```python
from build123d import *

# Parameters (mm, degrees)
BOSS_EXTRUDE2_DEPTH = 26
SKETCH5_R           = 1.6
CUT_EXTRUDE4_DEPTH  = 26
SKETCH6_R           = 1.6
CUT_EXTRUDE6_DEPTH  = 26


with BuildPart() as part:
    # Sketch1 → Boss-Extrude2 (new body)
    with BuildSketch(Plane(origin=(0, 0, 0), x_dir=(1, 0, 0), z_dir=(0, 1, 0))):
        Polygon((-24.25, 0), (24.25, 0), (24.25, -11), (39.25, -11), (39.25, -6), (29.25, -6), (29.25, 5), (5, 5), (5, 10), (-5, 10), (-5, 5), (-29.25, 5), (-29.25, -6), (-39.25, -6), (-39.25, -11), (-24.25, -11), align=None)
    extrude(amount=BOSS_EXTRUDE2_DEPTH)

    # Sketch5 → Cut-Extrude4 (cut)
    with BuildSketch(Plane.XZ):
        with Locations(Location((0, -5, 0), (0, 0, 270))):
            Circle(SKETCH5_R)
    extrude(amount=-CUT_EXTRUDE4_DEPTH, mode=Mode.SUBTRACT)

    # Sketch6 → Cut-Extrude6 (cut)
    with BuildSketch(Plane(origin=(0, 0, 6), x_dir=(-1, 0, 0), z_dir=(0, 0, -1))):
        with Locations((34.25, 19.5)):
            Circle(SKETCH6_R)
        with Locations((34.25, 6.5)):
            Circle(SKETCH6_R)
        with Locations((-34.25, 6.5)):
            Circle(SKETCH6_R)
        with Locations((-34.25, 19.5)):
            Circle(SKETCH6_R)
    extrude(amount=-CUT_EXTRUDE6_DEPTH, mode=Mode.SUBTRACT)


solid = part.part
```
Design review of the part built by this model. Coordinates are the model's own, in mm. A direction names the side the tool comes from. Give positions to 0.01 mm unless a question says otherwise; leave off trailing zeros. Write each loop counter-clockwise with the first axis right and the second up, starting at its lowest first coordinate (ties: lowest second). Pieces come first, ordered by that corner, then holes.
(1) Clearance check with flat-ended pins moving along their axes: pin 1 Ø3.5 at (x, y) = (34.25, 19.5) entering from +Z; pin 2 Ø5 at (x, y) = (32, 11.5) entering from -Z; pin 3 Ø3 at (x, y) = (-12.5, 7.5) entering from +Z; pin 4 Ø7.5 at (x, y) = (-13.5, 6.5) entering from -Z. State where each tip first meets the part, or that it passes through.
Checked values:
pin 1: stops at z = 11
pin 2: stops at z = 6
pin 3: stops at z = 0
pin 4: stops at z = -5
(2) Add section D-D (y = 3.5). Give the boundary of the cut face in (x, z), and give its area (3 significant figures).
Checked values:
outline: (-39.25, 6) - (-29.25, 6) - (-29.25, -5) - (-5, -5) - (-5, -10) - (5, -10) - (5, -5) - (29.25, -5) - (29.25, 6) - (39.25, 6) - (39.25, 11) - (24.25, 11) - (24.25, 0) - (-24.25, 0) - (-24.25, 11) - (-39.25, 11) - close; hole circle Ø3.2 at (0, -5)
area: 544 mm2
(3) Add section A-A (y = 19.5). Give the boundary of the cut face in (x, z), and give its area (3 significant figures).
Checked values:
outline: (-39.25, 6) - (-35.85, 6) - (-35.85, 11) - (-39.25, 11) - close; (-32.65, 6) - (-29.25, 6) - (-29.25, -5) - (-5, -5) - (-5, -10) - (5, -10) - (5, -5) - (29.25, -5) - (29.25, 6) - (32.65, 6) - (32.65, 11) - (24.25, 11) - (24.25, 0) - (-24.25, 0) - (-24.25, 11) - (-32.65, 11) - close; (35.85, 6) - (39.25, 6) - (39.25, 11) - (35.85, 11) - close; hole circle Ø3.2 at (0, -5)
area: 512 mm2
(4) Tool access review of faces 1 (the face through (-33.07, 20.58, 8.46)), 2 (the face through (17, 13, -5)), 3 (the face through (-5, 13, -8)), 4 (the face through (-24.25, 13, 6)): name each direction out of +Z, -Z, +X, -X, +Y, -Y from which nothing blocks a thin tool from reaching the whole face with its end or side.
Checked values:
face 1: +Z, -Z
face 2: -Z, +X, +Y, -Y
face 3: -Z, -X, +Y, -Y
face 4: +Z, +Y, -Y
(5) Mouldability with a two-part tool opening along Y and no side actions: class faces 5 (the face through (35.5, 5.5, 8.5)), 6 (the face through (-39.25, 13, 8)), 7 (the face through (3, 26, -1)), 8 (the face through (-33, 5.5, 8.5)) as +Y half, -Y half, draft (parallel to the pull), parting line (faces both ways), or undercut.
Checked values:
face 5: undercut
face 6: draft
face 7: +Y half
face 8: undercut
(6) Add section B-B (x = 34.25). Give the boundary of the cut face in (y, z).
Checked values:
outline: (0, 6) - (4.9, 6) - (4.9, 11) - (0, 11) - close; (8.1, 6) - (17.9, 6) - (17.9, 11) - (8.1, 11) - close; (21.1, 6) - (26, 6) - (26, 11) - (21.1, 11) - close
(7) Wall thickness on line 1 along Y through (x, z) = (34.25, 8); line 2 along X through (y, z) = (16.75, 2.5); line 3 along X through (y, z) = (5.5, 9.5): over which ranges is each line inside the solid? List them lowest first.
Checked values:
line 1: y = 0 to 4.9, 8.1 to 17.9, 21.1 to 26
line 2: x = -29.25 to -24.25, 24.25 to 29.25
line 3: x = -39.25 to -35.5, -33 to -24.25, 24.25 to 33, 35.5 to 39.25
(8) Add section C-C (x = 0). Give the boundary of the cut face in (y, z).
Checked values:
outline: (0, -10) - (26, -10) - (26, -6.6) - (0, -6.6) - close; (0, -3.4) - (26, -3.4) - (26, 0) - (0, 0) - close
